Input: part model. Units: mm. Frame: model coordinates. Face numbers are marked on the shaded views. A direction names the side the tool comes from. Give positions to 0.01 mm unless a question says otherwise; leave off trailing zeros. Order: outer loops, then holes, each group sorted by start corner. A loop starts at its lowest first (then second) coordinate and runs counter-clockwise, first axis right, second up. Notation, with made-up numbers: (80.25, 22.5) - (97.25, 22.5) arc R17 cw to (97.25, 45.5) - close; hole circle Ø9 at (53, 76). An arc over 180 degrees is marked (long way). Answer in a Markdown table with one row per item. Add a question column.
from build123d import *

# Parameters (mm, degrees)
BOSS_EXTRUDE3_DEPTH  = 125
SKETCH4_W            = 35
SKETCH4_H            = 35
BOSS_EXTRUDE4_DEPTH  = 20
CUT_EXTRUDE2_DEPTH   = 17
SKETCH6_W            = 35
SKETCH6_H            = 35
BOSS_EXTRUDE5_DEPTH  = 48
CUT_EXTRUDE3_START   = -20
CUT_EXTRUDE3_DEPTH   = 20
CUT_EXTRUDE4_DEPTH   = 26
FILLET1_R            = 12.7
FILLET2_R            = 2
SKETCH9_W            = 193
SKETCH9_H            = 35
BOSS_EXTRUDE6_DEPTH  = 2
SKETCH10_W           = 193
SKETCH10_H           = 35
BOSS_EXTRUDE7_DEPTH  = 2
SKETCH11_W           = 39
SKETCH11_H           = 35
BOSS_EXTRUDE8_DEPTH  = 2
SKETCH12_W           = 39
SKETCH12_H           = 35
BOSS_EXTRUDE9_DEPTH  = 2
SKETCH13_W           = 85
SKETCH13_H           = 17.5
CUT_EXTRUDE5_DEPTH   = 154.089026398
BOSS_EXTRUDE10_DEPTH = 4
BOSS_EXTRUDE11_DEPTH = 4
FILLET3_START        = -20
FILLET3_DEPTH        = 40
FILLET3_START_2      = -19.5
FILLET3_2_DEPTH      = 4
FILLET3_START_3      = 15.5
FILLET3_3_DEPTH      = 4


with BuildPart() as part:
    # Sketch1 → Boss-Extrude3 (new body)
    with BuildSketch(Plane.XY):
        with BuildLine():
            Line((0, -17.5), (-17.5, -17.5))
            Line((-17.5, -17.5), (-17.5, 0))
            Line((-17.5, 0), (-17.5, 17.5))
            Line((-17.5, 17.5), (-15.5, 17.5))
            Line((-15.5, 17.5), (-15.5, 0))
            ThreePointArc((-15.5, 0), (0, -15.5), (15.5, 0))
            Line((15.5, 0), (15.5, 17.5))
            Line((15.5, 17.5), (17.5, 17.5))
            Line((17.5, 17.5), (17.5, 0))
            Line((17.5, 0), (17.5, -17.5))
            Line((17.5, -17.5), (0, -17.5))
        make_face()
    extrude(amount=BOSS_EXTRUDE3_DEPTH)

    # Sketch4 → Boss-Extrude4 (add)
    with BuildSketch(Plane.XY.offset(125)):
        Rectangle(SKETCH4_W, SKETCH4_H)
    extrude(amount=BOSS_EXTRUDE4_DEPTH)

    # Sketch5 → Cut-Extrude2 (cut)
    with BuildSketch(Plane(origin=(0, 0, 125), x_dir=(-1, 0, 0), z_dir=(0, 0, -1))):
        with BuildLine():
            Line((-5, 0), (-5, 17.5))
            Line((-5, 17.5), (5, 17.5))
            Line((5, 17.5), (5, 0))
            ThreePointArc((5, 0), (0, -5), (-5, 0))
        make_face()
    extrude(amount=-CUT_EXTRUDE2_DEPTH, mode=Mode.SUBTRACT)

    # Sketch6 → Boss-Extrude5 (add)
    with BuildSketch(Plane(origin=(0, 0, 0), x_dir=(-1, 0, 0), z_dir=(0, 0, -1))):
        Rectangle(SKETCH6_W, SKETCH6_H)
    extrude(amount=BOSS_EXTRUDE5_DEPTH)

    # Sketch7 → Cut-Extrude3 (cut)
    with BuildSketch(Plane.XY.offset(CUT_EXTRUDE3_START)):
        with BuildLine():
            Line((-5, 0), (-5, 17.5))
            Line((-5, 17.5), (5, 17.5))
            Line((5, 17.5), (5, 0))
            ThreePointArc((5, 0), (0, -5), (-5, 0))
        make_face()
    extrude(amount=CUT_EXTRUDE3_DEPTH, mode=Mode.SUBTRACT)

    # Sketch8 → Cut-Extrude4 (cut)
    with BuildSketch(Plane.XY.offset(-20)):
        with BuildLine():
            Line((-13, 0), (-13, 27.339362416))
            Line((-13, 27.339362416), (13, 27.339362416))
            Line((13, 27.339362416), (13, 0))
            ThreePointArc((13, 0), (0, -13), (-13, 0))
        make_face()
    extrude(amount=-CUT_EXTRUDE4_DEPTH, mode=Mode.SUBTRACT)

    # Fillet1
    # the kernel refuses this fillet: 12.7 mm, written as the material it adds along each edge
    with BuildSketch(Plane(origin=(13, 17.5, -20), x_dir=(-1, 0, 0), z_dir=(0, -1, 0)), Plane(origin=(-13, 0, -20), x_dir=(1, 0, 0), z_dir=(0, 1, 0))) as fillet1_piece_1:
        with BuildLine():
            CenterArc((12.7, 11.798304963), FILLET1_R, 180, 68.279526527)
            Line((0, 11.798304963), (-0.254, 11.798304963))
            Line((-0.254, 11.798304963), (-0.254, 0))
            Line((-0.254, 0), (0, -0.254))
            ThreePointArc((0, -0.254), (4, -0.254), (7.906, -0.235966099))
            Line((7.906, -0.235966099), (8, 0))
        make_face()
    extrude(amount=17.5)
    with BuildSketch(Plane(origin=(0, 0, -20), x_dir=(1, 0, 0), z_dir=(0, 1, 0))) as fillet1_piece_2:
        with BuildLine():
            CenterArc((0.3, 11.798304963), FILLET1_R, 291.720473473, 68.279526527)
            Line((13, 11.798304963), (13.254, 11.798304963))
            Line((13.254, 11.798304963), (13.254, 0))
            Line((13.254, 0), (13, -0.254))
            ThreePointArc((13, -0.254), (9, -0.254), (5.094, -0.235966099))
            Line((5.094, -0.235966099), (5, 0))
        make_face()
    revolve(axis=Axis((0, 0, -20), (0, 0, -1)), revolution_arc=180)
    with BuildSketch(Plane(origin=(13, 17.5, -46), x_dir=(0, 0, 1), z_dir=(0, -1, 0))) as fillet1_piece_3:
        with BuildLine():
            CenterArc((FILLET1_R, FILLET1_R), FILLET1_R, 180, 90)
            Line((0, FILLET1_R), (-FILLET1_R * 0.02, FILLET1_R))
            Line((-FILLET1_R * 0.02, FILLET1_R), (-FILLET1_R * 0.02, -FILLET1_R * 0.02))
            Line((-FILLET1_R * 0.02, -FILLET1_R * 0.02), (FILLET1_R, -FILLET1_R * 0.02))
            Line((FILLET1_R, -FILLET1_R * 0.02), (FILLET1_R, 0))
        make_face()
    extrude(amount=17.5)
    with BuildSketch(Plane(origin=(0, 0, -46), x_dir=(1, 0, 0), z_dir=(0, 1, 0))) as fillet1_piece_4:
        with BuildLine():
            CenterArc((13 - FILLET1_R, -FILLET1_R), FILLET1_R, 0, 90)
            Line((13, -FILLET1_R), (13 + FILLET1_R * 0.02, -FILLET1_R))
            Line((13 + FILLET1_R * 0.02, -FILLET1_R), (13 + FILLET1_R * 0.02, FILLET1_R * 0.02))
            Line((13 + FILLET1_R * 0.02, FILLET1_R * 0.02), (13 - FILLET1_R, FILLET1_R * 0.02))
            Line((13 - FILLET1_R, FILLET1_R * 0.02), (13 - FILLET1_R, 0))
        make_face()
    revolve(axis=Axis((0, 0, -46), (0, 0, -1)), revolution_arc=180)
    with BuildSketch(Plane(origin=(-13, 0, -46), x_dir=(1, 0, 0), z_dir=(0, 1, 0))) as fillet1_piece_5:
        with BuildLine():
            CenterArc((FILLET1_R, -FILLET1_R), FILLET1_R, 90, 90)
            Line((0, -FILLET1_R), (-FILLET1_R * 0.02, -FILLET1_R))
            Line((-FILLET1_R * 0.02, -FILLET1_R), (-FILLET1_R * 0.02, FILLET1_R * 0.02))
            Line((-FILLET1_R * 0.02, FILLET1_R * 0.02), (FILLET1_R, FILLET1_R * 0.02))
            Line((FILLET1_R, FILLET1_R * 0.02), (FILLET1_R, 0))
        make_face()
    extrude(amount=17.5)

    # Fillet2
    fillet2_edges = [part.edges().sort_by_distance(p)[0] for p in [
        (0, -5, -20),
        (-5, 8.75, -20),
        (5, 8.75, -20),
        (0, -5, 0),
        (5, 8.75, 0),
        (-5, 8.75, 0),
    ]]
    fillet(fillet2_edges, radius=FILLET2_R)

    # Sketch9 → Boss-Extrude6 (add)
    with BuildSketch(Plane.ZY.offset(17.5)):
        with Locations((48.5, 0)):
            Rectangle(SKETCH9_W, SKETCH9_H)
    extrude(amount=BOSS_EXTRUDE6_DEPTH)

    # Sketch10 → Boss-Extrude7 (add)
    with BuildSketch(Plane(origin=(17.5, 0, 0), x_dir=(0, 0, -1), z_dir=(1, 0, 0))):
        with Locations((-48.5, 0)):
            Rectangle(SKETCH10_W, SKETCH10_H)
    extrude(amount=BOSS_EXTRUDE7_DEPTH)

    # Sketch11 → Boss-Extrude8 (add)
    with BuildSketch(Plane(origin=(0, 0, -48), x_dir=(-1, 0, 0), z_dir=(0, 0, -1))):
        Rectangle(SKETCH11_W, SKETCH11_H)
    extrude(amount=BOSS_EXTRUDE8_DEPTH)

    # Sketch12 → Boss-Extrude9 (add)
    with BuildSketch(Plane.XY.offset(145)):
        Rectangle(SKETCH12_W, SKETCH12_H)
    extrude(amount=BOSS_EXTRUDE9_DEPTH)

    # Sketch13 → Cut-Extrude5 (cut, through all)
    with BuildSketch(Plane(origin=(19.5, 0, 0), x_dir=(0, 0, -1), z_dir=(1, 0, 0))):
        with Locations((-62.5, 8.75)):
            Rectangle(SKETCH13_W, SKETCH13_H)
    extrude(amount=-CUT_EXTRUDE5_DEPTH, mode=Mode.SUBTRACT)

    # Sketch14 → Boss-Extrude10 (add)
    with BuildSketch(Plane(origin=(19.5, 0, 0), x_dir=(0, 0, -1), z_dir=(1, 0, 0))):
        Polygon((-105, 17.5), (-87.5, 0), (-105, 0), align=None)
        Polygon((-20, 0), (-20, 17.5), (-37.5, 0), align=None)
    extrude(amount=-BOSS_EXTRUDE10_DEPTH)

    # Sketch15 → Boss-Extrude11 (add)
    with BuildSketch(Plane.ZY.offset(19.5)):
        Polygon((20, 17.5), (37.5, 0), (20, 0), align=None)
        Polygon((105, 17.5), (87.5, 0), (105, 0), align=None)
    extrude(amount=-BOSS_EXTRUDE11_DEPTH)

    # Fillet3: read off the stored shape, not the designer's step
    # Fillet3 outline → Fillet3 (cut)
    with BuildSketch(Plane.YZ.offset(FILLET3_START)):
        with BuildLine():
            Line((17.5, 20), (16.035533906, 21.464466094))
            ThreePointArc((16.035533906, 21.464466094), (17.119397663, 19.84234935), (17.5, 17.928932188))
            Line((17.5, 17.928932188), (17.5, 20))
        make_face()
        with BuildLine():
            ThreePointArc((17.5, 107.071067812), (17.119397663, 105.15765065), (16.035533906, 103.535533906))
            Line((16.035533906, 103.535533906), (17.5, 105))
            Line((17.5, 105), (17.5, 107.071067812))
        make_face()
    extrude(amount=FILLET3_DEPTH, mode=Mode.SUBTRACT)

    # Fillet3 2 outline → Fillet3 2 (add)
    with BuildSketch(Plane.YZ.offset(FILLET3_START_2)):
        with BuildLine():
            Line((0, 87.5), (0, 85.428932188))
            ThreePointArc((0, 85.428932188), (0.380602337, 87.34234935), (1.464466094, 88.964466094))
            Line((1.464466094, 88.964466094), (0, 87.5))
        make_face()
        with BuildLine():
            Line((0, 37.5), (1.464466094, 36.035533906))
            ThreePointArc((1.464466094, 36.035533906), (0.380602337, 37.65765065), (0, 39.571067812))
            Line((0, 39.571067812), (0, 37.5))
        make_face()
    extrude(amount=FILLET3_2_DEPTH)

    # Fillet3 3 outline → Fillet3 3 (add)
    with BuildSketch(Plane.YZ.offset(FILLET3_START_3)):
        with BuildLine():
            Line((0, 87.5), (0, 85.428932188))
            ThreePointArc((0, 85.428932188), (0.380602337, 87.34234935), (1.464466094, 88.964466094))
            Line((1.464466094, 88.964466094), (0, 87.5))
        make_face()
        with BuildLine():
            Line((0, 37.5), (1.464466094, 36.035533906))
            ThreePointArc((1.464466094, 36.035533906), (0.380602337, 37.65765065), (0, 39.571067812))
            Line((0, 39.571067812), (0, 37.5))
        make_face()
    extrude(amount=FILLET3_3_DEPTH)


solid = part.part
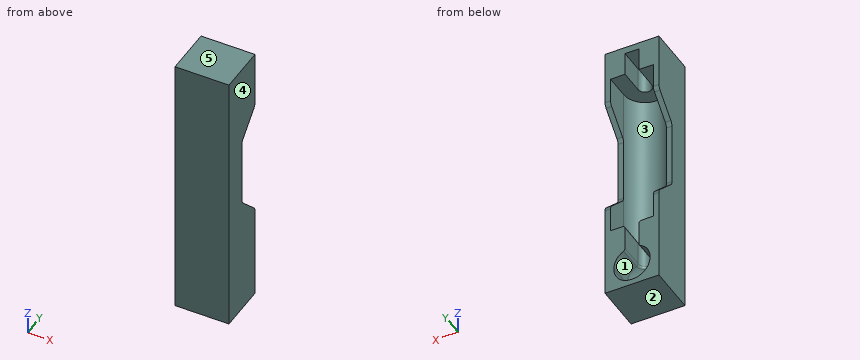
Q1. Pull-direction query (X, two-part tool) for the marked faces 3, 4 and 5; classes: +X half, -X half, draft (parallel to the pull), parting line (faces both ways), or undercut.
Q2. Access query for the marked faces 1 and 2. Directions: +Z, -Z, +X, -X, +Y, -Y. A direction counts if a zero-diameter tool reaches every point of the face in a straight line with its end or side. Return the directions, or none.
Q3. Section A-A, the plane z = 43.5. Return loops of the section in (x, y).
Q4. Line query: probe 1 along Z at (x, y) = (-10.5, -5); probe 2 along Z at (x, y) = (5, -3); probe 3 along X at (y, z) = (8, 18). Output: solid intervals per line, ascending.
Q5. Contact query for flat-ended pins moving along their axis: P1, Ø2, axis at x = -17, z = 65, coming from the +Y side; P2, Ø2, axis at x = 5.5, z = 36, coming from the +Y side. Output: stop coordinate, or through.
Computed:
| question | item | result |
|---|---|---|
| 1 | face 3 | undercut |
| 1 | face 4 | +X half |
| 1 | face 5 | draft |
| 2 | face 1 | +Y |
| 2 | face 2 | -Z, +X, -X, +Y, -Y |
| 3 | outline | (-19.5, -17.5) - (19.5, -17.5) - (19.5, 0) - (15.5, 0) arc R15.5 cw to (-15.5, 0) - (-19.5, 0) - close |
| 4 | probe 1 | z = -50 to -39.04, -26.06 to 0, 125 to 147 |
| 4 | probe 2 | z = -50 to -44.73, -20.34 to -0.38, 125 to 147 |
| 4 | probe 3 | x = -19.5 to -15.5, 15.5 to 19.5 |
| 5 | P1 | stops at y = 0 |
| 5 | P2 | stops at y = -14.07 |
